from build123d import *

# Parameters (mm, degrees)
SKETCH1_W           = 18
SKETCH1_H           = 16
SKETCH1_R           = 0.5
BOSS_EXTRUDE1_DEPTH = 5
FILLET2_R           = 1
FILLET3_R           = 1
FILLET4_R           = 1
FILLET5_R           = 1


with BuildPart() as part:
    # Sketch1 → Boss-Extrude1 (new body)
    with BuildSketch(Plane.XY):
        with Locations((9, 8)):
            Rectangle(SKETCH1_W, SKETCH1_H)
        with Locations((5.75, 4)):
            Circle(SKETCH1_R, mode=Mode.SUBTRACT)
        with Locations((7.25, 4)):
            Circle(SKETCH1_R, mode=Mode.SUBTRACT)
        with Locations((8.75, 4)):
            Circle(SKETCH1_R, mode=Mode.SUBTRACT)
        with Locations((10.25, 4)):
            Circle(SKETCH1_R, mode=Mode.SUBTRACT)
        with Locations((5.75, 12)):
            Circle(SKETCH1_R, mode=Mode.SUBTRACT)
        with Locations((6.25, 7.25)):
            Circle(SKETCH1_R, mode=Mode.SUBTRACT)
    extrude(amount=BOSS_EXTRUDE1_DEPTH)

    # Fillet2
    fillet2_edges = [part.edges().sort_by_distance(p)[0] for p in [
        (0, 0, 2.5),
    ]]
    fillet(fillet2_edges, radius=FILLET2_R)

    # Fillet3
    fillet3_edges = [part.edges().sort_by_distance(p)[0] for p in [
        (0, 16, 2.5),
    ]]
    fillet(fillet3_edges, radius=FILLET3_R)

    # Fillet4
    fillet4_edges = [part.edges().sort_by_distance(p)[0] for p in [
        (18, 16, 2.5),
    ]]
    fillet(fillet4_edges, radius=FILLET4_R)

    # Fillet5
    fillet5_edges = [part.edges().sort_by_distance(p)[0] for p in [
        (18, 0, 2.5),
    ]]
    fillet(fillet5_edges, radius=FILLET5_R)


solid = part.part
Design review of the part built by this model. Coordinates are the model's own, in mm. Round coordinates to 2 decimals unless told otherwise and drop trailing zeros. Order: outer loops, then holes, each group sorted by start corner. A loop starts at its lowest first (then second) coordinate and runs counter-clockwise, first axis right, second up.
1) For L1, parallel to Y at x = 8.75, z = 1.45; L2, parallel to Y at x = 5.5, z = 2.1; L3, parallel to X at y = 7, z = 1.05, list the stretches that pass through material, from the lowest coordinate up.
The answers:
L1: y = 0 to 3.5, 4.5 to 16
L2: y = 0 to 3.57, 4.43 to 11.57, 12.43 to 16
L3: x = 0 to 5.82, 6.68 to 18
2) Consider section B-B (y = 4). State the section outline as (x, z) points.
The answers:
outline: (0, 0) - (5.25, 0) - (5.25, 5) - (0, 5) - close; (6.25, 0) - (6.75, 0) - (6.75, 5) - (6.25, 5) - close; (7.75, 0) - (8.25, 0) - (8.25, 5) - (7.75, 5) - close; (9.25, 0) - (9.75, 0) - (9.75, 5) - (9.25, 5) - close; (10.75, 0) - (18, 0) - (18, 5) - (10.75, 5) - close
3) Consider section A-A (x = 7.25). State the section outline as (y, z) points.
The answers:
outline: (0, 0) - (3.5, 0) - (3.5, 5) - (0, 5) - close; (4.5, 0) - (16, 0) - (16, 5) - (4.5, 5) - close
4) Draft analysis for pull direction X (two halves, no side actions). For faces 1 (the flat face through (9, 16, 2)), 2 (the cylindrical face through (0.285, 0.301, 2.535)), 3 (the cylindrical face through (10.185, 4.496, 2.465)), state which applies: released by +X, released by -X, zero draft, split by the parting line, or undercut.
The answers:
face 1: zero draft
face 2: released by -X
face 3: undercut
5) Consider section C-C (z = 1.05). State the section outline as (x, y) points.
The answers:
outline: (0, 1) arc R1 ccw to (1, 0) - (17, 0) arc R1 ccw to (18, 1) - (18, 15) arc R1 ccw to (17, 16) - (1, 16) arc R1 ccw to (0, 15) - close; hole circle Ø1 at (5.75, 4); hole circle Ø1 at (5.75, 12); hole circle Ø1 at (6.25, 7.25); hole circle Ø1 at (7.25, 4); hole circle Ø1 at (8.75, 4); hole circle Ø1 at (10.25, 4)
